```python
from build123d import *

# Parameters (mm, degrees)
F0_R     = 11
F1_DEPTH = 8
F3_DEPTH = 4.5
F4_R     = 12.1301412178
F4_R_2   = 3.338839996
F5_DEPTH = 2
F7_SIZE  = 1
F8_W     = 2.0535623771
F8_H     = 2.0535623771
F9_DEPTH = 2
F10_R    = 0.5


# Not quite as in the source:
# - a fillet or chamfer that OpenCascade refuses, or shapes differently, is made with other operations: its cross-section is extruded or revolved along the edge and cut away or added


with BuildPart() as f1:
    # F0 (on Front) → F1 (new body)
    with BuildSketch(Plane.XZ):
        Circle(F0_R)
    extrude(amount=F1_DEPTH)

    # F2 (on face) → F3 (join)
    with BuildSketch(Plane.XZ.offset(8)):
        with BuildLine():
            Line((6.4951905284, 13.25), (-6.4951905284, 13.25))
            ThreePointArc((-6.4951905284, 13.25), (-7.4951905284, 12.9820508076), (-8.227241336, 12.25))
            Line((-8.227241336, 12.25), (-14.7224318643, 1))
            ThreePointArc((-14.7224318643, 1), (-14.9903810568, 0), (-14.7224318643, -1))
            Line((-14.7224318643, -1), (-8.227241336, -12.25))
            ThreePointArc((-8.227241336, -12.25), (-7.4951905284, -12.9820508076), (-6.4951905284, -13.25))
            Line((-6.4951905284, -13.25), (6.4951905284, -13.25))
            ThreePointArc((6.4951905284, -13.25), (7.4951905284, -12.9820508076), (8.227241336, -12.25))
            Line((8.227241336, -12.25), (14.7224318643, -1))
            ThreePointArc((14.7224318643, -1), (14.9903810568, 0), (14.7224318643, 1))
            Line((14.7224318643, 1), (8.227241336, 12.25))
            ThreePointArc((8.227241336, 12.25), (7.4951905284, 12.9820508076), (6.4951905284, 13.25))
        make_face()
    extrude(amount=F3_DEPTH)

    # F4 (on face) → F5 (join)
    with BuildSketch(Plane.XZ.offset(12.5)):
        Circle(F4_R)
        Circle(F4_R_2, mode=Mode.SUBTRACT)
    extrude(amount=F5_DEPTH)

    # F6: chamfer of 5 on 1 edges, made by hand


with BuildPart() as f6_tool2:
    # F6_s3 → F6_t4 (revolve)
    with BuildSketch(Plane.XY):
        Polygon((12.1301412178, -9.5), (7.1301412178, -14.5), (12.1301412178, -14.5), align=None)
    revolve(axis=Axis((0, -14.5, 0), (0, -1, 0)))

    split(bisect_by=Plane.XZ.offset(12.5), keep=Keep.TOP)


with BuildPart() as f1_1:
    add(f1.part)

    # F6_t1: cut F6_tool2
    add(f6_tool2.part, mode=Mode.SUBTRACT)

    # F7
    f7_edges = [f1_1.edges().sort_by_distance(p)[0] for p in [
        (-3.33884, -12.5, 0),
    ]]
    chamfer(f7_edges, length=F7_SIZE)

    # F8 (on face) → F9 (join)
    with BuildSketch(Plane.XZ.offset(12.5)):
        Rectangle(F8_W, F8_H)
    extrude(amount=F9_DEPTH)

    # F10
    f10_edges = [f1_1.edges().sort_by_distance(p)[0] for p in [
        (1.026781, -13.5, -1.026781),
        (-1.026781, -13.5, -1.026781),
        (-1.026781, -13.5, 1.026781),
        (1.026781, -13.5, 1.026781),
        (1.026781, -14.5, 0),
        (0, -14.5, 1.026781),
        (-1.026781, -14.5, 0),
        (0, -14.5, -1.026781),
    ]]
    fillet(f10_edges, radius=F10_R)


solid = f1_1.part
```
Here's how the part is built. I have some questions about the finished solid (model axes, mm). A direction names the side the tool comes from. Give positions to 0.01 mm unless a question says otherwise; leave off trailing zeros. Write each loop counter-clockwise with the first axis right and the second up, starting at its lowest first coordinate (ties: lowest second). Pieces come first, ordered by that corner, then holes. Notation, with made-up numbers: (44.5, 47) -> (68.5, 47) arc R15 cw to (68.5, 60) -> close; hole circle Ø10 at (2, 28.5). An arc over 180 degrees is marked (long way). Use one line per item in the form item = value.
1) Suppose I cut it at B-B (x = 0). Please give me the cut outline in (y, z), and give its area (3 significant figures).
Verdict:
outline = (-14.5, -7.13) -> (-12.5, -9.13) -> (-12.5, -13.25) -> (-8, -13.25) -> (-8, -11) -> (0, -11) -> (0, 11) -> (-8, 11) -> (-8, 13.25) -> (-12.5, 13.25) -> (-12.5, 9.13) -> (-14.5, 7.13) -> (-14.5, 3.34) -> (-13.5, 3.34) -> (-12.5, 2.34) -> (-12.5, 1.03) -> (-14, 1.03) arc R0.5 ccw to (-14.5, 0.53) -> (-14.5, -0.53) arc R0.5 ccw to (-14, -1.03) -> (-12.5, -1.03) -> (-12.5, -2.34) -> (-13.5, -3.34) -> (-14.5, -3.34) -> close
area = 319 mm2
2) I'm going to push flat-ended pins straight in: pin 1 (1.5 mm diameter, centred on x = 6.5, y = -3, fed in from -Z); pin 2 (8 mm diameter, centred on x = -10, y = -3, fed in from -Z); pin 3 (1 mm diameter, centred on y = -8, z = -9.5, fed in from +X). Where does each tip first touch, or does it pass through?
Verdict:
pin_1 = -9.38
pin_2 = -9.22
pin_3 = 10.1
3) Suppose I cut it at D-D (y = -5.5). Please give me the cut outline in (x, z).
Verdict:
outline = circle Ø22 at (0, 0)
4) We'd pull the mould along X, two halves only. Please class faces 1 (the face through (-14.99, -10.22, 0.01)), 2 (the face through (0, -13, 1.027)), 3 (the face through (11.43, -10.22, -6.7)): +X half, -X half, draft (parallel to the pull), parting line (faces both ways), or undercut.
Verdict:
face_1 = -X half
face_2 = undercut
face_3 = +X half
5) If I drill on L1, parallel to Z at x = 0, y = -13.75; L2, parallel to Z at x = 0, y = -14.05; L3, parallel to Y at x = 7.5, z = 9, over which ranges is the centre line in solid material (lowest first)? Write a range as [from, to].
Verdict:
L1 = [-7.88, -3.34], [-1.03, 1.03], [3.34, 7.88]
L2 = [-7.58, -3.34], [-1.02, 1.02], [3.34, 7.58]
L3 = [-12.5, -8]
6) Suppose I cut it at C-C (z = 0). Please give me the cut outline in (x, y), and give its area (3 significant figures).
Verdict:
outline = (-14.99, -12.5) -> (-9.13, -12.5) -> (-7.13, -14.5) -> (-3.34, -14.5) -> (-3.34, -13.5) -> (-2.34, -12.5) -> (-1.03, -12.5) -> (-1.03, -14) arc R0.5 ccw to (-0.53, -14.5) -> (0.53, -14.5) arc R0.5 ccw to (1.03, -14) -> (1.03, -12.5) -> (2.34, -12.5) -> (3.34, -13.5) -> (3.34, -14.5) -> (7.13, -14.5) -> (9.13, -12.5) -> (14.99, -12.5) -> (14.99, -8) -> (11, -8) -> (11, 0) -> (-11, 0) -> (-11, -8) -> (-14.99, -8) -> close
area = 335 mm2
7) Suppose I cut it at A-A (y = -9). Please give me the cut outline in (x, z), and give its area (3 significant figures).
Verdict:
outline = (-14.72, -1) -> (-8.23, -12.25) arc R2 ccw to (-6.5, -13.25) -> (6.5, -13.25) arc R2 ccw to (8.23, -12.25) -> (14.72, -1) arc R2 ccw to (14.72, 1) -> (8.23, 12.25) arc R2 ccw to (6.5, 13.25) -> (-6.5, 13.25) arc R2 ccw to (-8.23, 12.25) -> (-14.72, 1) arc R2 ccw to start
area = 607 mm2
8) On a 3-axis mill with a long thin cutter (end or side, diameter ignored), from which of +Z, -Z, +X, -X, +Y, -Y can I reach the whole of each face in a straight line? I mean faces 4 (the face through (-8, -8, 8)), 5 (the face through (0, -13, -1.027)), 6 (the face through (-2, -14.5, -3)). Say none if no direction works.
Verdict:
face_4 = +Y
face_5 = -Y
face_6 = +Z, -Z, +X, -X, -Y
